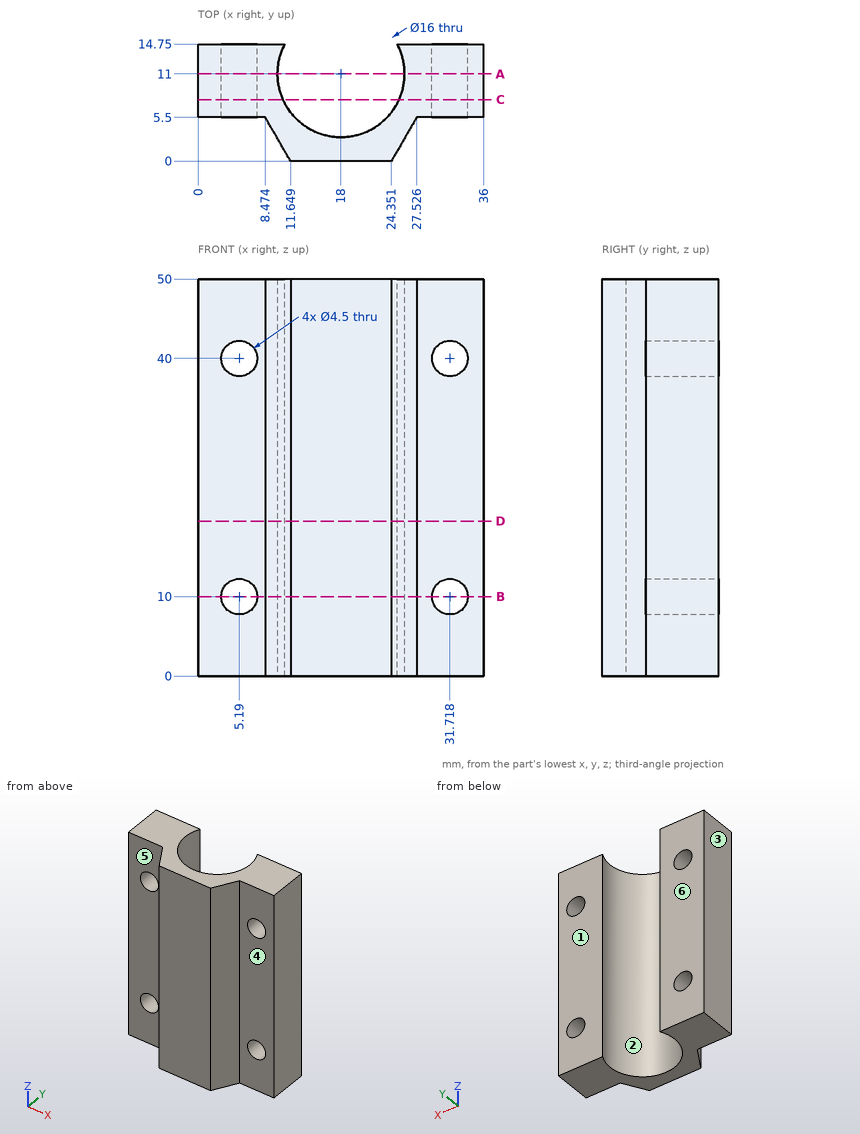
Drawing for the job (mm, zero at the part's lowest x, y, z). A direction names the side the tool comes from. Coordinates: 2 decimals unless noted, no trailing zeros. Loops run counter-clockwise (first coordinate to the right, second up) from the corner with the lowest first, then second, coordinate; pieces in that order, holes last. Notation, with made-up numbers: (48, 69) - (104, 69) arc R17 cw to (104, 86) - close; hole circle Ø8 at (79.5, -5.75). An arc over 180 degrees is marked (long way). Return JSON: item names as keys, results as strings.
1. Band-saw the part on B-B (z = 10). Give the cut face in (x, y).
Result:
{"outline": "(0, 5.5) - (2.94, 5.5) - (2.94, 14.75) - (0, 14.75) - close; (7.44, 5.5) - (8.47, 5.5) - (11.65, 0) - (24.35, 0) - (27.53, 5.5) - (29.47, 5.5) - (29.47, 14.75) - (25.07, 14.75) arc R8 cw (long way) to (10.93, 14.75) - (7.44, 14.75) - close; (33.97, 5.5) - (36, 5.5) - (36, 14.75) - (33.97, 14.75) - close"}
2. Mould opens along Y. For the marked faces 1, 2, 3 and 4 say: released by +Y, released by -Y, zero draft, split by the parting line, or undercut.
Result:
{"face 1": "released by +Y", "face 2": "undercut", "face 3": "zero draft", "face 4": "released by -Y"}
3. Probe L1, parallel to Z at x = 31.5, y = 12.5; L2, parallel to X at y = 11.25, z = 40; L3, parallel to X at y = 11, z = 35.5. List the from-to ranges inside material, lowest first. Write a range as from..to.
Result:
{"L1": "z = 0..7.76, 12.24..37.76, 42.24..50", "L2": "x = 0..2.94, 7.44..10, 26..29.47, 33.97..36", "L3": "x = 0..10, 26..36"}
4. Drop flat-ended pins along their axis: pin 1 (4 mm diameter, centred on x = 4, z = 14, fed in from -Y); pin 2 (2.5 mm diameter, centred on x = 31.72, z = 10, fed in from +Y); pin 3 (4 mm diameter, centred on x = 13, z = 32.5, fed in from +Y) (1 decimal); pin 4 (9.5 mm diameter, centred on x = 31.5, z = 34.5, fed in from -Y) (1 decimal). Give the stop position or say it passes through.
Result:
{"pin 1": "stops at y = 5.5", "pin 2": "passes through", "pin 3": "stops at y = 7.1", "pin 4": "stops at y = 4.2"}
5. Band-saw the part on D-D (z = 19.5). Give the cut face in (x, y).
Result:
{"outline": "(0, 5.5) - (8.47, 5.5) - (11.65, 0) - (24.35, 0) - (27.53, 5.5) - (36, 5.5) - (36, 14.75) - (25.07, 14.75) arc R8 cw (long way) to (10.93, 14.75) - (0, 14.75) - close"}
6. Band-saw the part on C-C (y = 7.75). Give the cut face in (x, z).
Result:
{"outline": "(0, 0) - (10.69, 0) - (10.69, 50) - (0, 50) - close; (25.31, 0) - (36, 0) - (36, 50) - (25.31, 50) - close; hole circle Ø4.5 at (5.19, 10); hole circle Ø4.5 at (5.19, 40); hole circle Ø4.5 at (31.72, 10); hole circle Ø4.5 at (31.72, 40)"}
7. 3-axis set-ups, long thin cutter, end or side, ignore diameter. For the marked faces 5 and 6: which of +Z, -Z, +X, -X, +Y, -Y reach the whole face in a straight line?
Result:
{"face 5": "+Z, -Z, -X, -Y", "face 6": "+Z, -Z, +X, -X, +Y"}
8. Band-saw the part on A-A (y = 11). Give the cut face in (x, z).
Result:
{"outline": "(0, 0) - (10, 0) - (10, 50) - (0, 50) - close; (26, 0) - (36, 0) - (36, 50) - (26, 50) - close; hole circle Ø4.5 at (5.19, 10); hole circle Ø4.5 at (5.19, 40); hole circle Ø4.5 at (31.72, 10); hole circle Ø4.5 at (31.72, 40)"}
